Geometry: final body of the model. Coordinates: model frame, mm. Give positions to 0.01 mm unless a question says otherwise; leave off trailing zeros. Write each loop counter-clockwise with the first axis right and the second up, starting at its lowest first coordinate (ties: lowest second). Pieces come first, ordered by that corner, then holes. Notation, with made-up numbers: M -24.75,46.25 L -11.75,46.25 A27 ccw -11.75,81.25 Z; hole C 88,28 d8. An arc over 180 degrees is marked long. Use a Markdown table: item, result. Add a question column.
(1) Cut plane C-C (x = 1.4). Output: boundary loops of the cut face in (y, z), plus the area to 3 significant figures.
(2) Cut plane D-D (x = -0.7). Output: boundary loops of the cut face in (y, z), plus the area to 3 significant figures.
(3) Material intervals for L1, parallel to X at y = -9, z = 8.5; L2, parallel to Y at x = 1.55, z = 0; L3, parallel to Z at x = -1, y = 0, sorted ascending.
(4) Pin query (flat end, axial travel): pin 1 Ø3 at (x, z) = (-1.5, -8.5) entering from -Y; pin 2 Ø1 at (x, z) = (1, -3) entering from +Y; pin 3 Ø2 at (x, z) = (0, -5.5) entering from -Y. Return the tip coordinate at first contact, or that it passes through.
(5) Cut plane A-A (y = 0). Output: boundary loops of the cut face in (x, z), plus the area to 3 significant figures.
(6) Draft query along X for faces 1 (the flat face through (2.1, 7.35, 9.2)), 2 (the flat face through (-2.1, 7.35, 9.2)), 3 (the flat face through (-2.5, 0, 8)), 4 (the cylindrical face through (-1.32, -7.493, 0.33)). Return one class per face: released by +X, released by -X, zero draft, split by the parting line, or undercut.
Solid Edge part; units mm, degrees
sketch "Sketch1" plane through (0, 0, 0) normal (0, 0, 1) x (1, 0, 0)
  line L0 (-2.5, 12.5) -> (-2.5, 7.5)
  line L1 (-2.5, 7.5) -> (-0.1732, 7.5)
  line L2 (-0.1732, 7.5) -> (0, 7.8)
  line L3 (0, 7.8) -> (0.1732, 7.5)
  line L4 (0.1732, 7.5) -> (2.5, 7.5)
  line L5 (2.5, 7.5) -> (2.5, 12.5)
  line L6 (2.5, 12.5) -> (2.1, 12.5)
  line L7 (2.1, 12.5) -> (2.1, 11.6)
  arc A0 (2.1, 11.6) -> (-2.1, 11.6) centre (0, 11.6) cw
  line L8 (-2.1, 11.6) -> (-2.1, 12.5)
  line L9 (-2.1, 12.5) -> (-2.5, 12.5)
revolve "RevolvedProtrusion1" add sketch "Sketch1" angle 360 about axis through (2.5, 0, 0) along (-1, 0, 0)
properties material "Steel"
Answer list:
| question | item | result |
|---|---|---|
| 1 | outline | C 0,0 d20.07; hole C 0,0 d15 |
| 1 | area | 140 mm² |
| 2 | outline | C 0,0 d19.24; hole C 0,0 d15 |
| 2 | area | 114 mm² |
| 3 | L1 | -2.5 to -2.1, 2.1 to 2.5 |
| 3 | L2 | -10.18 to -7.5, 7.5 to 10.18 |
| 3 | L3 | -9.75 to -7.5, 7.5 to 9.75 |
| 4 | pin 1 | y = -10.27 |
| 4 | pin 2 | y = 9.7 |
| 4 | pin 3 | y = -8.37 |
| 5 | outline | M -2.5,-12.5 L -2.1,-12.5 L -2.1,-11.6 A2.1 cw 2.1,-11.6 L 2.1,-12.5 L 2.5,-12.5 L 2.5,-7.5 L 0.17,-7.5 L 0,-7.8 L -0.17,-7.5 L -2.5,-7.5 Z; M -2.5,7.5 L -0.17,7.5 L 0,7.8 L 0.17,7.5 L 2.5,7.5 L 2.5,12.5 L 2.1,12.5 L 2.1,11.6 A2.1 cw -2.1,11.6 L -2.1,12.5 L -2.5,12.5 Z |
| 5 | area | 28.5 mm² |
| 6 | face 1 | undercut |
| 6 | face 2 | undercut |
| 6 | face 3 | released by -X |
| 6 | face 4 | zero draft |
